Geometry check sheet. Reference: the model listing, model coordinates, mm. A direction names the side the tool comes from. Coordinates: 2 decimals unless noted, no trailing zeros. Write each loop counter-clockwise with the first axis right and the second up, starting at its lowest first coordinate (ties: lowest second). Pieces come first, ordered by that corner, then holes. Notation, with made-up numbers: (62, 70) -> (69, 70) arc R26 ccw to (69, 84) -> close; hole circle Ø8 at (10.25, 14.25). An arc over 180 degrees is marked (long way). Answer in a Markdown table with one row per item. Add a question column.
Q1. Section check A-A, the plane z = 8. Record the boundary of the cut face in (x, y).
Q2. Thickness scan on line 1 (Y direction, x = -24.5, z = 7); line 2 (Z direction, x = -2.5, y = -26.15); line 3 (Z direction, x = -8.85, y = -26.15). Record the ranges inside material, lowest first.
Q3. Section check C-C, the plane z = 41.5. Record the boundary of the cut face in (x, y), and give its area (3 significant figures).
Q4. Tool access check on faces 4 (the face through (-8.965, -24.616, 42.515)), 5 (the face through (-15, -26, 10)), 6 (the face through (0, -26, 30)), 7 (the face through (-5, -26, 60)), 8 (the face through (-26, -20.989, 5)). Record the directions out of +Z, -Z, +X, -X, +Y, -Y that give a thin tool (end or side, any length) a straight path to the whole face; none if there is none.
Q5. Release check for a two-part mould opening along Y. For faces 1 (the face through (-30, -42, 5)), 2 (the face through (-7.9, -21, 48)), 3 (the face through (-5.07, -50.87, 58.5)) record: pulls with the +Y half, pulls with the -Y half, needs draft (parallel to the pull), parting line crosses it, or undercut.
Q6. Gauge pin test, flat ends, axial feed: P1, Ø7, axis at y = -29, z = 49, coming from the -X side; P2, Ø15, axis at y = -33.5, z = 32.5, coming from the -X side; P3, Ø10, axis at x = -24, y = -18.5, coming from the +Z side. Record the tip position at first contact, or that the pin passes through.
Q7. Section check B-B, the plane y = -18. Record the boundary of the cut face in (x, z).
```python
from build123d import *

# Parameters (mm, degrees)
F1_DEPTH  = 52.3
F2_R      = 5
F3_DEPTH  = 12.5
F4_R      = 5
F5_R      = 5
F6_R      = 7.07449
F6_R_2    = 5
F8_DEPTH  = 2.1
F10_DEPTH = 25


with BuildPart() as f1:
    # F0 (on Front) → F1 (new body)
    with BuildSketch(Plane.XZ):
        Polygon((0, 0), (0, 60), (-10, 60), (-10, 10), (-30, 10), (-30, 0), align=None)
    extrude(amount=F1_DEPTH)

    # F2 (on face) → F3 (cut, symmetric)
    with BuildSketch(Plane.YZ):
        with Locations((-26.15, 49.421053)):
            Circle(F2_R)
    extrude(amount=F3_DEPTH, both=True, mode=Mode.SUBTRACT)

    # F4
    f4_edges = [f1.edges().sort_by_distance(p)[0] for p in [
        (-5, -52.3, 60),
    ]]
    fillet(f4_edges, radius=F4_R)

    # F5
    f5_edges = [f1.edges().sort_by_distance(p)[0] for p in [
        (-5, 0, 60),
    ]]
    fillet(f5_edges, radius=F5_R)

    # F6 (on face) → F8 (cut)
    with BuildSketch(Plane(origin=(-10, 0, 0), x_dir=(0, -1, 0), z_dir=(-1, 0, 0))):
        with Locations((26.15, 49.421053)):
            Circle(F6_R)
        with Locations((26.15, 49.421053)):
            Circle(F6_R_2, mode=Mode.SUBTRACT)
    extrude(amount=-F8_DEPTH, mode=Mode.SUBTRACT)

    # F9 (on face) → F10 (cut)
    with BuildSketch(Plane.XY.offset(10)):
        with BuildLine():
            ThreePointArc((-22.569968, -31.228698), (-18.247574, -30.169685), (-16.337931, -26.15))
            ThreePointArc((-16.337931, -26.15), (-18.038064, -22.310553), (-22.023625, -20.988769))
            ThreePointArc((-22.023625, -20.988769), (-26.701406, -25.873729), (-22.569968, -31.228698))
        make_face()
        with BuildLine():
            ThreePointArc((-22.569968, -31.228698), (-26.701406, -25.873729), (-22.023625, -20.988769))
            Line((-22.023625, -20.988769), (-30, -20.988769))
            Line((-30, -20.988769), (-30, -31.228698))
            Line((-30, -31.228698), (-22.569968, -31.228698))
        make_face()
    extrude(amount=-F10_DEPTH, mode=Mode.SUBTRACT)


solid = f1.part
```
Calculated:
| question | item | result |
|---|---|---|
| 1 | outline | (-30, -52.3) -> (0, -52.3) -> (0, 0) -> (-30, 0) -> (-30, -20.99) -> (-22.02, -20.99) arc R5.19 cw (long way) to (-22.57, -31.23) -> (-30, -31.23) -> close |
| 2 | line 1 | y = -52.3 to -31.23, -20.99 to 0 |
| 2 | line 2 | z = 0 to 44.42, 54.42 to 60 |
| 2 | line 3 | z = 0 to 42.35, 56.5 to 60 |
| 3 | outline | (-10, -52.3) -> (0, -52.3) -> (0, 0) -> (-10, 0) -> close |
| 3 | area | 523 mm² |
| 4 | face 4 | -X |
| 4 | face 5 | +Z, -X, +Y, -Y |
| 4 | face 6 | +Z, -Z, +X, +Y, -Y |
| 4 | face 7 | +Z, +X, -X, +Y, -Y |
| 4 | face 8 | +Z, -Z, -X |
| 5 | face 1 | needs draft |
| 5 | face 2 | undercut |
| 5 | face 3 | pulls with the -Y half |
| 6 | P1 | stops at x = -7.9 |
| 6 | P2 | stops at x = -10 |
| 6 | P3 | stops at z = 10 |
| 7 | outline | (-30, 0) -> (0, 0) -> (0, 60) -> (-10, 60) -> (-10, 10) -> (-30, 10) -> close |
